```python
from build123d import *

# Parameters (mm, degrees)
F0_W     = 12.5
F0_H     = 5
F1_DEPTH = 17
F2_DEPTH = 2
F3_W     = 3
F3_H     = 20.822813987
F3_H_2   = 20
F4_DEPTH = 25
F5_W     = 17
F5_H     = 12.5
F5_W_2   = 10.3
F5_H_2   = 10.3
F6_DEPTH = 5


with BuildPart() as f1:
    # F0 (on Right) → F1 (new body)
    with BuildSketch(Plane.YZ):
        with BuildLine():
            ThreePointArc((6.25, 7), (0, 13.25), (-6.25, 7))
            Line((-6.25, 7), (-4.6188021535, 7))
            Line((-4.6188021535, 7), (-2.3094010768, 11))
            Line((-2.3094010768, 11), (2.3094010768, 11))
            Line((2.3094010768, 11), (4.6188021535, 7))
            Line((4.6188021535, 7), (6.25, 7))
        make_face()
        Polygon((-6.25, 7), (-6.25, 0), (6.25, 0), (6.25, 7), (4.6188021535, 7), (2.3094010768, 3), (-2.3094010768, 3), (-4.6188021535, 7), align=None)
        with BuildLine():
            Line((-2.5, 7), (-4.6188021535, 7))
            Line((-4.6188021535, 7), (-2.3094010768, 3))
            Line((-2.3094010768, 3), (2.3094010768, 3))
            Line((2.3094010768, 3), (4.6188021535, 7))
            Line((4.6188021535, 7), (2.5, 7))
            ThreePointArc((2.5, 7), (0, 4.5), (-2.5, 7))
        make_face()
        with BuildLine():
            Line((-2.3094010768, 11), (-4.6188021535, 7))
            Line((-4.6188021535, 7), (-2.5, 7))
            ThreePointArc((-2.5, 7), (0, 9.5), (2.5, 7))
            Line((2.5, 7), (4.6188021535, 7))
            Line((4.6188021535, 7), (2.3094010768, 11))
            Line((2.3094010768, 11), (-2.3094010768, 11))
        make_face()
        with Locations((0, -2.5)):
            Rectangle(F0_W, F0_H)
    extrude(amount=F1_DEPTH)

    # F0 (on Right) → F2 (cut)
    with BuildSketch(Plane.YZ):
        with BuildLine():
            Line((-2.3094010768, 11), (-4.6188021535, 7))
            Line((-4.6188021535, 7), (-2.5, 7))
            ThreePointArc((-2.5, 7), (0, 9.5), (2.5, 7))
            Line((2.5, 7), (4.6188021535, 7))
            Line((4.6188021535, 7), (2.3094010768, 11))
            Line((2.3094010768, 11), (-2.3094010768, 11))
        make_face()
        with BuildLine():
            Line((-2.5, 7), (-4.6188021535, 7))
            Line((-4.6188021535, 7), (-2.3094010768, 3))
            Line((-2.3094010768, 3), (2.3094010768, 3))
            Line((2.3094010768, 3), (4.6188021535, 7))
            Line((4.6188021535, 7), (2.5, 7))
            ThreePointArc((2.5, 7), (0, 4.5), (-2.5, 7))
        make_face()
    extrude(amount=F2_DEPTH, mode=Mode.SUBTRACT)

    # F3 (on Top) → F4 (cut)
    with BuildSketch(Plane.XY):
        with Locations((6, -0.3987241719)):
            Rectangle(F3_W, F3_H)
        with Locations((12, -1.1113596391)):
            Rectangle(F3_W, F3_H_2)
    extrude(amount=F4_DEPTH, mode=Mode.SUBTRACT)

    # F5 (on face) → F6 (join)
    with BuildSketch(Plane(origin=(0, 0, -5), x_dir=(1, 0, 0), z_dir=(0, 0, -1))):
        with Locations((8.5, 0)):
            Rectangle(F5_W, F5_H)
        with Locations((8.5, 0)):
            Rectangle(F5_W_2, F5_H_2, mode=Mode.SUBTRACT)
    extrude(amount=F6_DEPTH)


solid = f1.part
```
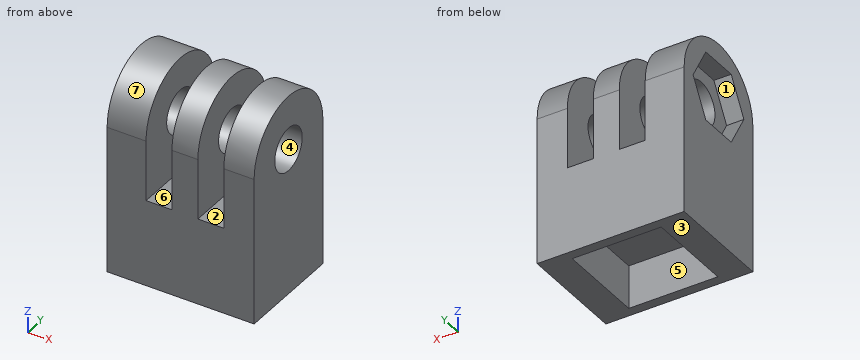
Can you work these out from the model? Positions are in its coordinate system, mm. Face numbers are marked on the shaded views. A direction names the side the tool comes from. Coordinates: 2 decimals unless noted, no trailing zeros. Loops run counter-clockwise (first coordinate to the right, second up) from the corner with the lowest first, then second, coordinate; pieces in that order, holes last. Notation, with made-up numbers: (-36.75, 77) - (7.25, 77) arc R20 cw to (7.25, 94) - close; hole circle Ø5 at (11.5, -20.5). An arc over 180 degrees is marked (long way). Answer as CSV lines item,"result". Start each with the question number.
1) I need wall thicknesses on line 1 (X direction, y = -4.25, z = 5.75); line 2 (X direction, y = 2.5, z = 6.5); line 3 (X direction, y = 3, z = -6). Which ranges of each line are inside material? Lowest first, please. Write a range as from..to.
2) For pin 1 (3 mm diameter, centred on y = 0, z = 7, fed in from +X); pin 2 (6 mm diameter, centred on y = 0, z = 7, fed in from -X); pin 3 (3.5 mm diameter, centred on x = 12, y = -1.5, fed in from +Z), each with a flat end and sliding along its axis, tell me the tip position at first contact or that it passes through.
3) Suppose I cut it at D-D (y = 3.75). Please give me the cut outline in (x, z).
4) Thinking about a two-plate mould opening in Z: for the marked faces 1, 2, 3 and 4, which applies, pulls with the +Z half, pulls with the -Z half, needs draft (parallel to the pull), parting line crosses it, or undercut?
5) Which directions (+Z, -Z, +X, -X, +Y, -Y) give clear straight access to the entire face, cutting with the end or side of a thin tool? Please do the marked faces 5, 6 and 7.
6) Suppose I cut it at A-A (y = 0). Count the separate pieces of the cut face and the enclosed holes in it, plus the area to 3 significant figures.
7) Suppose I cut it at C-C (x = 15.25). Please give me the cut outline in (y, z), plus the area to 3 significant figures.
8) Suppose I cut it at B-B (x = 5). Please give me the cut outline in (y, z).
Check result:
1,line 1,"x = 0..4.5, 7.5..10.5, 13.5..17"
1,line 2,"x = 2..4.5, 7.5..10.5, 13.5..17"
1,line 3,"x = 0..3.35, 13.65..17"
2,pin 1,"passes through"
2,pin 2,"stops at x = 2"
2,pin 3,"stops at z = 13.22"
3,outline,"(0, -10) - (3.35, -10) - (3.35, -5) - (13.65, -5) - (13.65, -10) - (17, -10) - (17, 12) - (13.5, 12) - (13.5, 0) - (10.5, 0) - (10.5, 12) - (7.5, 12) - (7.5, 0) - (4.5, 0) - (4.5, 12) - (0, 12) - (0, 8.5) - (2, 8.5) - (2, 5.5) - (0, 5.5) - close"
4,face 1,"undercut"
4,face 2,"pulls with the +Z half"
4,face 3,"pulls with the -Z half"
4,face 4,"undercut"
5,face 5,"-Z"
5,face 6,"+Z, +Y, -Y"
5,face 7,"+Z, +X, -X"
6,separate pieces,"4"
6,enclosed holes,"0"
6,area,"203 mm²"
7,outline,"(-6.25, -10) - (6.25, -10) - (6.25, 7) arc R6.25 ccw to (-6.25, 7) - close; hole circle Ø5 at (0, 7)"
7,area,"254 mm²"
8,outline,"(-6.25, -10) - (-5.15, -10) - (-5.15, -5) - (5.15, -5) - (5.15, -10) - (6.25, -10) - (6.25, 0) - (-6.25, 0) - close"
